Verification items for the finished model (mm, model axes). A direction names the side the tool comes from. Round coordinates to 2 decimals unless told otherwise and drop trailing zeros. Order: outer loops, then holes, each group sorted by start corner. A loop starts at its lowest first (then second) coordinate and runs counter-clockwise, first axis right, second up. Notation, with made-up numbers: M -34,47 L 5,47 A28 ccw 5,80 Z; hole C 26.25,88 d6. An arc over 180 degrees is marked long. One line per item, written item: value. Start each with the question number.
from build123d import *

# Parameters (mm, degrees)
SKETCH1_W                 = 94.5
SKETCH1_H                 = 70
BOSS_EXTRUDE1_DEPTH       = 45
F_3_0MM_DOWEL_HOLE1_D     = 3
F_3_0MM_DOWEL_HOLE1_DEPTH = 30
F_3_0MM_DOWEL_HOLE1_TIP   = 0.901290929
SKETCH7_W                 = 55
SKETCH7_H                 = 28
CUT_EXTRUDE2_DEPTH        = 20
SHELL2_START              = 2
SHELL2_DEPTH              = 43
SHELL2_START_2            = 22
SHELL2_2_OUTLINE_W        = 59
SHELL2_2_OUTLINE_H        = 31
SHELL2_2_DEPTH            = 23
SHELL2_3_DEPTH            = 11.868454444
CUT_EXTRUDE3_DEPTH        = 1.5
BOSS_EXTRUDE9_DEPTH       = 11
F_3_0MM_DOWEL_HOLE3_D     = 3
F_3_0MM_DOWEL_HOLE3_DEPTH = 10
F_3_0MM_DOWEL_HOLE3_TIP   = 0.901290929
SKETCH15_R                = 3.5
CUT_EXTRUDE4_DEPTH        = 3
SKETCH30_W                = 10.076322372
SKETCH30_H                = 8
BOSS_EXTRUDE5_DEPTH       = 20
SKETCH31_W                = 15
SKETCH31_H                = 10.554348819
BOSS_EXTRUDE6_DEPTH       = 20
F_3_0MM_DOWEL_HOLE4_D     = 3
F_3_0MM_DOWEL_HOLE4_DEPTH = 41
F_3_0MM_DOWEL_HOLE4_TIP   = 0.901290929
SKETCH27_W                = 12
SKETCH27_H                = 6
CUT_EXTRUDE5_DEPTH        = 30
SKETCH33_R                = 4
BOSS_EXTRUDE7_DEPTH       = 15
SKETCH34_R                = 2
CUT_EXTRUDE6_DEPTH        = 30
FILLET1_R                 = 4
FILLET2_R                 = 4
FILLET3_R                 = 2


with BuildPart() as part:
    # Sketch1 → Boss-Extrude1 (new body)
    with BuildSketch(Plane(origin=(0, 0, 0), x_dir=(1, 0, 0), z_dir=(0, 1, 0))):
        Rectangle(SKETCH1_W, SKETCH1_H)
    extrude(amount=BOSS_EXTRUDE1_DEPTH)

    # Ø3.0mm Dowel Hole1
    with Locations(Plane(origin=(-43.75, 45, -31.5), x_dir=(0, 0, 1), z_dir=(0, 1, 0))):
        with Locations((0, 0), (0, 87.5), (63, 87.5), (63, 0)):
            Hole(F_3_0MM_DOWEL_HOLE1_D / 2, depth=F_3_0MM_DOWEL_HOLE1_DEPTH)
            with Locations((0, 0, -(F_3_0MM_DOWEL_HOLE1_DEPTH + F_3_0MM_DOWEL_HOLE1_TIP / 2))):  # 118° drill point
                Cone(0, F_3_0MM_DOWEL_HOLE1_D / 2, F_3_0MM_DOWEL_HOLE1_TIP, mode=Mode.SUBTRACT)

    # Sketch7 → Cut-Extrude2 (cut)
    with BuildSketch(Plane.XZ):
        with Locations((0, 18)):
            Rectangle(SKETCH7_W, SKETCH7_H)
    extrude(amount=-CUT_EXTRUDE2_DEPTH, mode=Mode.SUBTRACT)

    # Shell2: read off the stored shape, not the designer's step
    # Shell2 outline → Shell2 (cut)
    with BuildSketch(Plane(origin=(0, 0, 0), x_dir=(1, 0, 0), z_dir=(0, 1, 0)).offset(SHELL2_START)):
        with BuildLine():
            Line((-45.25, 28.33772234), (-45.25, -28.33772234))
            ThreePointArc((-45.25, -28.33772234), (-41.275126266, -29.025126266), (-40.58772234, -33))
            Line((-40.58772234, -33), (-29.5, -33))
            Line((-29.5, -33), (-29.5, -2))
            Line((-29.5, -2), (29.5, -2))
            Line((29.5, -2), (29.5, -33))
            Line((29.5, -33), (40.58772234, -33))
            ThreePointArc((40.58772234, -33), (41.275126266, -29.025126266), (45.25, -28.33772234))
            Line((45.25, -28.33772234), (45.25, 28.33772234))
            ThreePointArc((45.25, 28.33772234), (41.275126266, 29.025126266), (40.58772234, 33))
            Line((40.58772234, 33), (-40.58772234, 33))
            ThreePointArc((-40.58772234, 33), (-41.275126266, 29.025126266), (-45.25, 28.33772234))
        make_face()
    extrude(amount=SHELL2_DEPTH, mode=Mode.SUBTRACT)

    # Shell2 2 outline → Shell2 2 (cut)
    with BuildSketch(Plane(origin=(0, 0, 0), x_dir=(1, 0, 0), z_dir=(0, 1, 0)).offset(SHELL2_START_2)):
        with Locations((0, -17.5)):
            Rectangle(SHELL2_2_OUTLINE_W, SHELL2_2_OUTLINE_H)
    extrude(amount=SHELL2_2_DEPTH, mode=Mode.SUBTRACT)

    # Shell2 3 outline → Shell2 3 (cut)
    with BuildSketch(Plane(origin=(0, 0, 0), x_dir=(1, 0, 0), z_dir=(0, 1, 0)).offset(SHELL2_START)):
        with BuildLine():
            Line((-45.25, -28.33772234), (-45.25, -33))
            Line((-45.25, -33), (-40.58772234, -33))
            ThreePointArc((-40.58772234, -33), (-41.275126266, -29.025126266), (-45.25, -28.33772234))
        make_face()
        with BuildLine():
            Line((-45.25, 33), (-45.25, 28.33772234))
            ThreePointArc((-45.25, 28.33772234), (-41.275126266, 29.025126266), (-40.58772234, 33))
            Line((-40.58772234, 33), (-45.25, 33))
        make_face()
        with BuildLine():
            Line((45.25, 33), (40.58772234, 33))
            ThreePointArc((40.58772234, 33), (41.275126266, 29.025126266), (45.25, 28.33772234))
            Line((45.25, 28.33772234), (45.25, 33))
        make_face()
        with BuildLine():
            ThreePointArc((45.25, -28.33772234), (41.275126266, -29.025126266), (40.58772234, -33))
            Line((40.58772234, -33), (45.25, -33))
            Line((45.25, -33), (45.25, -28.33772234))
        make_face()
    extrude(amount=SHELL2_3_DEPTH, mode=Mode.SUBTRACT)

    # Shell2 4 outline → Shell2 4 (revolve)
    with BuildSketch(Plane(origin=(-43.75, 0, 31.5), x_dir=(1, 0, 0), z_dir=(0, 0, 1))):
        Polygon((0, 13.868454444), (0, 11.765442277), (3.5, 13.868454444), align=None)
    revolve(axis=Axis((-43.75, 0, 31.5), (0, 1, 0)))

    # Shell2 5 outline → Shell2 5 (revolve)
    with BuildSketch(Plane(origin=(43.75, 0, 31.5), x_dir=(1, 0, 0), z_dir=(0, 0, 1))):
        Polygon((0, 13.868454444), (0, 11.765442277), (3.5, 13.868454444), align=None)
    revolve(axis=Axis((43.75, 0, 31.5), (0, 1, 0)))

    # Shell2 6 outline → Shell2 6 (revolve)
    with BuildSketch(Plane(origin=(43.75, 0, -31.5), x_dir=(1, 0, 0), z_dir=(0, 0, 1))):
        Polygon((0, 13.868454444), (0, 11.765442277), (3.5, 13.868454444), align=None)
    revolve(axis=Axis((43.75, 0, -31.5), (0, 1, 0)))

    # Shell2 7 outline → Shell2 7 (revolve)
    with BuildSketch(Plane(origin=(-43.75, 0, -31.5), x_dir=(1, 0, 0), z_dir=(0, 0, 1))):
        Polygon((0, 13.868454444), (0, 11.765442277), (3.5, 13.868454444), align=None)
    revolve(axis=Axis((-43.75, 0, -31.5), (0, 1, 0)))

    # Sketch8 → Cut-Extrude3 (cut)
    with BuildSketch(Plane.XZ):
        with BuildLine():
            Line((27.5, 25), (27.5, 11))
            ThreePointArc((27.5, 11), (34.5, 18), (27.5, 25))
        make_face()
        with BuildLine():
            ThreePointArc((-27.5, 25), (-34.5, 18), (-27.5, 11))
            Line((-27.5, 11), (-27.5, 25))
        make_face()
    extrude(amount=-CUT_EXTRUDE3_DEPTH, mode=Mode.SUBTRACT)

    # Sketch36 → Boss-Extrude9 (add)
    with BuildSketch(Plane.XZ.offset(-1.5)):
        with BuildLine():
            Line((-27.5, 25), (-27.5, 11))
            ThreePointArc((-27.5, 11), (-34.5, 18), (-27.5, 25))
        make_face()
        with BuildLine():
            Line((27.5, 25), (27.5, 11))
            ThreePointArc((27.5, 11), (34.5, 18), (27.5, 25))
        make_face()
    extrude(amount=-BOSS_EXTRUDE9_DEPTH)

    # Ø3.0mm Dowel Hole3
    with Locations(Plane(origin=(31.2, 1.5, 18), x_dir=(0, 0, -1), z_dir=(0, -1, 0))):
        with Locations((0, 0), (0, -62.4)):
            Hole(F_3_0MM_DOWEL_HOLE3_D / 2, depth=F_3_0MM_DOWEL_HOLE3_DEPTH)
            with Locations((0, 0, -(F_3_0MM_DOWEL_HOLE3_DEPTH + F_3_0MM_DOWEL_HOLE3_TIP / 2))):  # 118° drill point
                Cone(0, F_3_0MM_DOWEL_HOLE3_D / 2, F_3_0MM_DOWEL_HOLE3_TIP, mode=Mode.SUBTRACT)

    # Sketch15 → Cut-Extrude4 (cut)
    with BuildSketch(Plane.ZY.offset(-27.5)):
        with Locations(Location((15.383017002, 17, 0), (0, 0, 58.997280866))):
            Circle(SKETCH15_R)
    extrude(amount=-CUT_EXTRUDE4_DEPTH, mode=Mode.SUBTRACT)

    # Sketch30 → Boss-Extrude5 (add)
    with BuildSketch(Plane(origin=(0, 2, 0), x_dir=(1, 0, 0), z_dir=(0, 1, 0))):
        with Locations((34.538161186, -29)):
            Rectangle(SKETCH30_W, SKETCH30_H)
        with Locations((-34.538161186, -29)):
            Rectangle(SKETCH30_W, SKETCH30_H)
    extrude(amount=BOSS_EXTRUDE5_DEPTH)

    # Sketch31 → Boss-Extrude6 (add)
    with BuildSketch(Plane(origin=(0, 2, 0), x_dir=(1, 0, 0), z_dir=(0, 1, 0))):
        with Locations((37.75, 27.722825591)):
            Rectangle(SKETCH31_W, SKETCH31_H)
    extrude(amount=BOSS_EXTRUDE6_DEPTH)

    # Ø3.0mm Dowel Hole4
    with Locations(Plane(origin=(36.25, 45, 28), x_dir=(0, 0, 1), z_dir=(0, 1, 0))):
        with Locations((0, 0), (0.35318171, -72.224429626), (-56, 0)):
            Hole(F_3_0MM_DOWEL_HOLE4_D / 2, depth=F_3_0MM_DOWEL_HOLE4_DEPTH)
            with Locations((0, 0, -(F_3_0MM_DOWEL_HOLE4_DEPTH + F_3_0MM_DOWEL_HOLE4_TIP / 2))):  # 118° drill point
                Cone(0, F_3_0MM_DOWEL_HOLE4_D / 2, F_3_0MM_DOWEL_HOLE4_TIP, mode=Mode.SUBTRACT)

    # Sketch27 → Cut-Extrude5 (cut)
    with BuildSketch(Plane(origin=(0, 0, -35), x_dir=(-1, 0, 0), z_dir=(0, 0, -1))):
        with Locations((27.5, 37)):
            Rectangle(SKETCH27_W, SKETCH27_H)
    extrude(amount=-CUT_EXTRUDE5_DEPTH, mode=Mode.SUBTRACT)

    # Sketch33 → Boss-Extrude7 (add)
    with BuildSketch(Plane.XY.offset(35)):
        with Locations(Location((0, 35, 0), (0, 0, 180))):
            Circle(SKETCH33_R)
    extrude(amount=BOSS_EXTRUDE7_DEPTH)

    # Sketch34 → Cut-Extrude6 (cut)
    with BuildSketch(Plane.XY.offset(50)):
        with Locations((0, 35)):
            Circle(SKETCH34_R)
    extrude(amount=-CUT_EXTRUDE6_DEPTH, mode=Mode.SUBTRACT)

    # Fillet1
    fillet1_edges = [part.edges().sort_by_distance(p)[0] for p in [
        (4, 35, 35),
    ]]
    fillet(fillet1_edges, radius=FILLET1_R)

    # Fillet2
    fillet2_edges = [part.edges().sort_by_distance(p)[0] for p in [
        (47.25, 22.5, 35),
        (-47.25, 22.5, 35),
        (-47.25, 22.5, -35),
        (47.25, 22.5, -35),
    ]]
    fillet(fillet2_edges, radius=FILLET2_R)

    # Fillet3
    fillet3_edges = [part.edges().sort_by_distance(p)[0] for p in [
        (0, 0, 35),
        (47.25, 0, 0),
        (-47.25, 0, 0),
        (0, 0, -35),
        (46.078427125, 0, -33.828427125),
        (46.078427125, 0, 33.828427125),
        (-46.078427125, 0, -33.828427125),
        (-46.078427125, 0, 33.828427125),
    ]]
    fillet(fillet3_edges, radius=FILLET3_R)


solid = part.part
1. Section check C-C (z = -9). Record the cut outline in (x, y).
2. Section check A-A (x = 0). Record the cut outline in (y, z).
3. Scan lines: line 1 along Z through (x, y) = (15, 27); line 2 along X through (y, z) = (37, 4); line 3 along Z through (x, y) = (-37, 7). Record each from-to range of solid material in increasing order.
4. Tool access check on faces 4 (the face through (-44.66, 29.79, -30.31)), 5 (the face through (0, 45, 34)), 6 (the face through (0, 10, 4)). Record the directions out of +Z, -Z, +X, -X, +Y, -Y that give a thin tool (end or side, any length) a straight path to the whole face; none if there is none.
5. Section check D-D (y = 8.5). Give the number of separate pieces and of enclosed holes in the cut face, and give its area (3 significant figures).
6. Depth check by flat-ended pin: pin 1 (1 mm diameter, centred on y = 38, z = -34, fed in from -X); pin 2 (6 mm diameter, centred on x = 13, y = 14, fed in from +Z); pin 3 (2.5 mm diameter, centred on x = 32.5, z = 17, fed in from +Y). Enter the tip coordinate at first touch or a pass-through.
7. Section check B-B (x = 9.5). Record the cut outline in (y, z), and give its area (3 significant figures).
8. Draft check along Z on faces 1 (the face through (-1, 0, -8)), 2 (the face through (-46.047, 23.801, 33.859)), 3 (the face through (-27.5, 10, 18)). Enter one of: released by +Z, released by -Z, zero draft, split by the parting line, or undercut.
Geometry check:
1. outline: M -47.25,2 A2 ccw -45.25,0 L 45.25,0 A2 ccw 47.25,2 L 47.25,45 L 45.25,45 L 45.25,2 L -45.25,2 L -45.25,45 L -47.25,45 Z
2. outline: M 0,-33 A2 ccw 2,-35 L 45,-35 L 45,-33 L 2,-33 L 2,2 L 22,2 L 22,33 L 33,33 L 33,50 L 31,50 L 31,39 A4 cw 27,35 L 2,35 A2 ccw 0,33 L 0,32 L 20,32 L 20,4 L 0,4 Z; M 37,33 L 45,33 L 45,35 L 43,35 A4 cw 39,39 L 39,50 L 37,50 Z
3. line 1: z = -35 to -33, 33 to 35
3. line 2: x = -47.25 to -45.25, 45.25 to 47.25
3. line 3: z = -35 to -33, 25 to 27.26, 29.45 to 35
4. face 4: +Y
4. face 5: +Z, -Z, +X, -X, +Y
4. face 6: -Y
5. separate pieces: 1
5. enclosed holes: 7
5. area: 1,300 mm²
6. pin 1: stops at x = -46.37
6. pin 2: stops at z = 35
6. pin 3: stops at y = 12.5
7. outline: M 0,-33 A2 ccw 2,-35 L 45,-35 L 45,-33 L 2,-33 L 2,2 L 22,2 L 22,33 L 45,33 L 45,35 L 2,35 A2 ccw 0,33 L 0,32 L 20,32 L 20,4 L 0,4 Z
7. area: 370 mm²
8. face 1: zero draft
8. face 2: released by +Z
8. face 3: undercut
